Autodesk Inventor part; units mm, degrees
ref_plane "YZ Plane" through (0, 0, 0) normal (1, 0, 0) x (0, 1, 0)
ref_plane "XZ Plane" through (0, 0, 0) normal (0, 1, 0) x (-1, 0, 0)
ref_plane "XY Plane" through (0, 0, 0) normal (0, 0, 1) x (1, 0, 0)
sketch "Sketch1" plane through (0, 0, 0) normal (0, 1, 0) x (-1, 0, 0)
  line L0 (0, 0) -> (46, 0) construction
  line L1 (46, 0) -> (46, -46) construction
  line L2 (46, -46) -> (0, -46) construction
  line L3 (0, -46) -> (0, 0) construction
  circle A0 centre (46, -46) radius 1.5
  circle A1 centre (46, 0) radius 1.5
  circle A2 centre (0, 0) radius 1.5
  circle A3 centre (0, -46) radius 1.5
  line L4 (23, 0) -> (23, -46) construction
  line L5 (-8, 8) -> (54, 8)
  line L6 (54, 8) -> (54, -54)
  line L7 (54, -54) -> (-8, -54)
  line L8 (-8, -54) -> (-8, 8)
  line L9 (-8, 8) -> (54, -54) construction
  line L10 (54, 8) -> (-8, -54) construction
  point P0 (23, -23)
  dimension "d0" = 46
  dimension "d1" = 46
  dimension "d2" = 3
  dimension "d3" = 3
  dimension "d4" = 3
  dimension "d5" = 3
  dimension "d6" = 8
  dimension "d7" = 8
extrude "Extrusion1" add sketch "Sketch1" along normal blind 5
sketch "Sketch2" plane through (0, 5, 0) normal (0, 1, 0) x (1, 0, 0)
  line L0 (-54, -8) -> (8, -8)
  line L1 (-54, -8) -> (-114, -8)
  line L2 (-114, -8) -> (-114, 54)
  line L3 (-114, 54) -> (-54, 54)
  line L4 (-54, 54) -> (-54, -8)
  line L5 (8, 54) -> (-54, 54)
  point P0 (0, 0)
  dimension "d10" = 60
extrude "Extrusion2" add sketch "Sketch2" against normal blind 5
sketch "Sketch3" plane through (0, 5, 0) normal (0, 1, 0) x (1, 0, 0)
  circle A0 centre (0, 46) radius 1.5
  circle A1 centre (-46, 46) radius 1.5
  line L0 (0, 46) -> (-46, 46) construction
  line L1 (-23, 46) -> (-23, 0) construction
  line L2 (-1.5, 44.5) -> (-44.5, 44.5)
  line L3 (-44.5, 44.5) -> (-44.5, 1.5)
  line L4 (-44.5, 1.5) -> (-1.5, 1.5)
  line L5 (-1.5, 1.5) -> (-1.5, 44.5)
  line L6 (-1.5, 44.5) -> (-44.5, 1.5) construction
  line L7 (-44.5, 44.5) -> (-1.5, 1.5) construction
  line L8 (-114, -8) -> (8, -8)
  point P0 (0, 0)
  point P1 (-23, 23)
  dimension "d14" = 43
  dimension "d15" = 43
extrude "Extrusion3" cut sketch "Sketch3" against normal blind 5 contours L5 L4 L3 L2
fillet "Fillet1" radius 1 4 edges at (-44.5, 2.5, -44.5) (-44.5, 2.5, -1.5) (-1.5, 2.5, -1.5) (-1.5, 2.5, -44.5)
sketch "Sketch4" plane through (0, 5, 0) normal (0, 1, 0) x (1, 0, 0)
  circle A0 centre (-108, 40) radius 1.5
  circle A1 centre (-108, -2) radius 1.5
  line L0 (-114, -8) -> (8, -8)
  line L1 (-114, 54) -> (-114, -8)
  line L2 (8, 54) -> (-114, 54)
  circle A2 centre (-59, -2) radius 1.5
  circle A3 centre (-59, 48) radius 1.5
  circle A4 centre (-66, -2) radius 1.5
  circle A5 centre (-66, 48) radius 1.5
  line L3 (-59, -2) -> (-59, 48) construction
  line L4 (-66, 46.5) -> (-59, 46.5)
  line L5 (-66, 49.5) -> (-59, 49.5)
  line L6 (-66, -3.5) -> (-59, -3.5)
  line L7 (-66, -0.5) -> (-59, -0.5)
  line L8 (-66, -2) -> (-66, 48) construction
  line L9 (-59, -2) -> (-66, -2) construction
  line L10 (-59, 48) -> (-66, 48) construction
  point P0 (0, 0)
  dimension "d19" = 6
  dimension "d20" = 3
  dimension "d21" = 6
  dimension "d23" = 3
  dimension "d24" = 6
  dimension "d25" = 14
  dimension "d26" = 3
  dimension "d27" = 3
  dimension "d28" = 50
  dimension "d29" = 6
  dimension "d32" = 7
  dimension "d33" = 3
  dimension "d34" = 3
  dimension "d35" = 7
  dimension "d36" = 42
extrude "Extrusion4" cut sketch "Sketch4" against normal blind 5
fillet "Fillet2" [suppressed]
sketch "Sketch5" plane through (0, 5, 0) normal (0, 1, 0) x (1, 0, 0)
  line L0 (-114, -8) -> (8, -8)
  line L1 (8, 54) -> (-54, 54)
  line L2 (-54, 54) -> (-54, -8)
  line L3 (-54, -8) -> (8, -8)
  line L4 (8, -8) -> (8, 54)
  line L5 (-114, 54) -> (-114, -8)
  point P0 (0, 0)
  point P1 (8, -8)
  dimension "d42" = 60
extrude "Extrusion5" cut sketch "Sketch5" against normal blind 10
sketch "Sketch6" plane through (0, 5, 0) normal (0, 1, 0) x (1, 0, 0)
  circle A0 centre (-95, 13) radius 5
  circle A1 centre (-108, 40) radius 1.5
  circle A2 centre (-85, 13) radius 5.099
  line L0 (-95, 18) -> (-84, 18)
  line L1 (-95, 8) -> (-85.0506, 7.9012)
  point P0 (0, 0)
  dimension "d45" = 27
  dimension "d46" = 13
  dimension "d47" = 10
  dimension "d48" = 10
extrude "Extrusion6" cut sketch "Sketch6" against normal blind 10 contours A0 A2 | L0 A2 A0 | A0 A2 L1 | A2 L0 A0 | A0 A2
fillet "Fillet3" radius 2 2 edges at (-54, 2.5, 8) (-54, 2.5, -54)
properties part number "Electronics cover"
Geometry check sheet. Reference: the model listing, model coordinates, mm. A direction names the side the tool comes from. Give positions to 0.01 mm unless a question says otherwise; leave off trailing zeros. Write each loop counter-clockwise with the first axis right and the second up, starting at its lowest first coordinate (ties: lowest second). Pieces come first, ordered by that corner, then holes.
1) Thickness scan on line 1 (Z direction, x = -60, y = 2.5); line 2 (X direction, y = 1.3, z = 2); line 3 (Z direction, x = -108, y = 2.05). Record the ranges inside material, lowest first.
Values follow:
line 1: z = -54 to -49.5, -46.5 to 0.5, 3.5 to 8
line 2: x = -114 to -109.5, -106.5 to -67.5, -57.5 to -54
line 3: z = -54 to -41.5, -38.5 to 0.5, 3.5 to 8
2) Cross-section at D-D (x = -88.5). Record the boundary of the cut face in (y, z), plus the area to 3 significant figures.
Values follow:
outline: (0, -54) - (5, -54) - (5, -18) - (0, -18) - close; (0, -7.94) - (5, -7.94) - (5, 8) - (0, 8) - close
area: 260 mm2
3) Go/stop test with flat-tipped pins: pin 1 Ø8 at (x, z) = (-104.5, -40) entering from -Y; pin 2 Ø1.8 at (x, z) = (-108, -40) entering from +Y. Record where each tip stops, or that it passes through.
Values follow:
pin 1: stops at y = 0
pin 2: passes through
4) Cross-section at A-A (z = 2). Record the boundary of the cut face in (x, y), plus the area to 3 significant figures.
Values follow:
outline: (-114, 0) - (-109.5, 0) - (-109.5, 5) - (-114, 5) - close; (-106.5, 0) - (-67.5, 0) - (-67.5, 5) - (-106.5, 5) - close; (-57.5, 0) - (-54, 0) - (-54, 5) - (-57.5, 5) - close
area: 235 mm2
5) Release check for a two-part mould opening along X. For faces 1 (the face through (-63, 3, 3.5)), 2 (the face through (-85, 2, -54)), 3 (the face through (-114, 3, -23)), 4 (the face through (-54, 3, -23)) record: released by +X, released by -X, zero draft, split by the parting line, or undercut.
Values follow:
face 1: undercut
face 2: zero draft
face 3: released by -X
face 4: released by +X
6) Set-up check for faces 5 (the face through (-100, 3, -13)), 6 (the face through (-84, 0, -23)): record each of +Z, -Z, +X, -X, +Y, -Y from which the full face is reachable in a straight line by a thin tool's end or side.
Values follow:
face 5: +Y, -Y
face 6: +Z, -Z, +X, -X, -Y
7) Cross-section at B-B (x = -108). Record the boundary of the cut face in (y, z).
Values follow:
outline: (0, -54) - (5, -54) - (5, -41.5) - (0, -41.5) - close; (0, -38.5) - (5, -38.5) - (5, 0.5) - (0, 0.5) - close; (0, 3.5) - (5, 3.5) - (5, 8) - (0, 8) - close
8) Cross-section at C-C (z = -48). Record the boundary of the cut face in (x, y), plus the area to 3 significant figures.
Values follow:
outline: (-114, 0) - (-67.5, 0) - (-67.5, 5) - (-114, 5) - close; (-57.5, 0) - (-54, 0) - (-54, 5) - (-57.5, 5) - close
area: 250 mm2
